from build123d import *

# Parameters (mm, degrees)
CUT_EXTRUDE_1798_DEPTH   = 103.8
CUT_EXTRUDE_3_REACH      = 141.642
CUT_EXTRUDE_3_END_RADIUS = 48


with BuildPart() as part:
    # Эскиз1 → Повернуть1 (revolve)
    with BuildSketch(Plane.XY):
        Polygon((21.7, 60), (31.7, 60), (31.7, 70), (33.2, 70), (35.7, 45.751288694), (43.350635095, 32.5), (45, 32.5), (45, 2.5), (48, 2.5), (48, 32.5), (50, 32.5), (50, 0), (42, 0), (42, 24.839368606), align=None)
    revolve(axis=Axis((0, 4, 0), (0, -1, 0)))

    # Эскиз3 → Cut-Extrude 1798 (cut, symmetric)
    with BuildSketch(Plane.XY):
        with BuildLine():
            Line((3.700961894, 9.781798364), (5, 12.031798364))
            Line((5, 12.031798364), (6.299038106, 9.781798364))
            ThreePointArc((6.299038106, 9.781798364), (5, 7.531798364), (3.700961894, 9.781798364))
        make_face()
        with BuildLine():
            Line((-3.700961894, 9.781798364), (-5, 12.031798364))
            Line((-5, 12.031798364), (-6.299038106, 9.781798364))
            ThreePointArc((-6.299038106, 9.781798364), (-5, 7.531798364), (-3.700961894, 9.781798364))
        make_face()
    extrude(amount=CUT_EXTRUDE_1798_DEPTH, both=True, mode=Mode.SUBTRACT)

    # Вырез-Вытянуть3: up to this cylinder (the profile starts outside it)
    cut_extrude_3_end = Plane(origin=(0, 9.031798, 0), z_dir=(0, -1, 0)) * Cylinder(CUT_EXTRUDE_3_END_RADIUS, 380.284, mode=Mode.PRIVATE)
    # Эскиз4 → Вырез-Вытянуть3 (cut, up to the surface)
    with BuildSketch(Plane.XY.offset(-60), mode=Mode.PRIVATE) as cut_extrude_3_sk1:
        with BuildLine():
            Line((-5, 10.531798364), (5, 10.531798364))
            ThreePointArc((5, 10.531798364), (6.5, 9.031798364), (5, 7.531798364))
            Line((5, 7.531798364), (-5, 7.531798364))
            ThreePointArc((-5, 7.531798364), (-6.5, 9.031798364), (-5, 10.531798364))
        make_face()
    cut_extrude_3_tool1 = extrude(cut_extrude_3_sk1.sketch, amount=CUT_EXTRUDE_3_REACH, mode=Mode.PRIVATE) - cut_extrude_3_end
    cut_extrude_3 = cut_extrude_3_tool1.solids().sort_by_distance((0, 9.031798, -60))[0]
    add(cut_extrude_3, mode=Mode.SUBTRACT)

    # Зеркальное отражение1: Вырез-Вытянуть3 across plane
    add(cut_extrude_3.mirror(Plane.XY), mode=Mode.SUBTRACT)


solid = part.part
Input: part model. Units: mm. Frame: model coordinates. A direction names the side the tool comes from. Round coordinates to 2 decimals unless told otherwise and drop trailing zeros. Write each loop counter-clockwise with the first axis right and the second up, starting at its lowest first coordinate (ties: lowest second). Pieces come first, ordered by that corner, then holes.
1) Reachability of faces 1 (the cylindrical face through (19.38, 12.59, -37.26)), 2 (the cylindrical face through (-5.044, 7.532, -43.155)), 3 (the flat face through (19, 32.5, 45)) from +Z, -Z, +X, -X, +Y, -Y: full face, straight path, thin tool, end or side. Return the list, or none.
2) Cut plane B-B (y = 22). Return the cut outline in (x, z).
3) Cut plane A-A (z = 0). Return the cut outline in (x, y), then the cut area to 3 significant figures.
4) Contact query for flat-ended pins moving along their axis: P1, Ø6, axis at y = 12, z = -28.5, coming from the +X side; P2, Ø10, axis at y = 38.5, z = -31.5, coming from the +X side; P3, Ø1.8, axis at x = 5, y = 9.03, coming from the -Z side; P4, Ø2.5, axis at x = 2.5, z = 49, coming from the +Y side. Output: stop coordinate, or through.
5) Ray query, L1, parallel to Z at x = 0, y = 13.5; L2, parallel to Z at x = -9, y = 16.5; L3, parallel to X at y = 13, z = 4.5. Return the intervals inside material, ascending.
6) Draft query along X for faces 4 (the flat face through (-27, 70, -17)), 5 (the cylindrical face through (-5.044, 7.532, 43.202)), 6 (the conical face through (-34.157, 60.4, 1.503)). Return one class per face: pulls with the +X half, pulls with the -X half, needs draft (parallel to the pull), parting line crosses it, or undercut.
7) Cut plane C-C (x = 0). Count the separate pieces of the cut face and the enclosed holes in it, then the cut area to 3 significant figures.
Geometry says:
1. face 1: -Y
1. face 2: +Z, -Z
1. face 3: +Y
2. outline: circle Ø100 at (0, 0); circle Ø90 at (0, 0); hole circle Ø96 at (0, 0); hole circle Ø84 at (0, 0)
3. outline: (-50, 0) - (-42, 0) - (-42, 24.84) - (-21.7, 60) - (-31.7, 60) - (-31.7, 70) - (-33.2, 70) - (-35.7, 45.75) - (-43.35, 32.5) - (-45, 32.5) - (-45, 2.5) - (-48, 2.5) - (-48, 32.5) - (-50, 32.5) - close; (21.7, 60) - (42, 24.84) - (42, 0) - (50, 0) - (50, 32.5) - (48, 32.5) - (48, 2.5) - (45, 2.5) - (45, 32.5) - (43.35, 32.5) - (35.7, 45.75) - (33.2, 70) - (31.7, 70) - (31.7, 60) - close
3. area: 828 mm2
4. P1: stops at x = 43.01
4. P2: stops at x = 31.25
4. P3: passes through
4. P4: stops at y = 32.5
5. L1: z = -50 to -48, -45 to -42, 42 to 45, 48 to 50
5. L2: z = -49.18 to -47.15, -44.09 to -41.02, 41.02 to 44.09, 47.15 to 49.18
5. L3: x = -49.8 to -47.79, -44.77 to -41.76, 41.76 to 44.77, 47.79 to 49.8
6. face 4: needs draft
6. face 5: undercut
6. face 6: parting line crosses it
7. separate pieces: 4
7. enclosed holes: 0
7. area: 816 mm2
